Autodesk Inventor part; units mm, degrees
ref_plane "YZ Plane" through (0, 0, 0) normal (1, 0, 0) x (0, 1, 0)
ref_plane "XZ Plane" through (0, 0, 0) normal (0, 1, 0) x (-1, 0, 0)
ref_plane "XY Plane" through (0, 0, 0) normal (0, 0, 1) x (1, 0, 0)
sketch "Sketch2" plane through (0, 0, 0) normal (0, 0, 1) x (1, 0, 0)
  line L0 (-197.082, 197.082) -> (0, 278.716)
  line L1 (0, 278.716) -> (197.082, 197.082)
  line L2 (197.082, 197.082) -> (278.716, 0)
  line L3 (278.716, 0) -> (197.082, -197.082)
  line L4 (197.082, -197.082) -> (0, -278.716)
  line L5 (0, -278.716) -> (-197.082, -197.082)
  line L6 (-197.082, -197.082) -> (-278.716, 0)
  line L7 (-278.716, 0) -> (-197.082, 197.082)
  circle A0 centre (0, 0) radius 90
  dimension "d23" = 515
  dimension "d26" = 180
extrude "Plate1" add sketch "Sketch2" against normal blind 3
sketch "Sketch4" plane through (0, 0, 0) normal (0, 0, 1) x (1, 0, 0)
  circle A0 centre (0, 110) radius 6.25
  circle A1 centre (0, 0) radius 90
  circle A2 centre (0, 0) radius 110 construction
  dimension "d28" = 220
  dimension "d16" = 12.5
extrude "Extrusion1" cut sketch "Sketch4" against normal up to surface (3 mm away) contours A0
pattern_circular "Circular Pattern1" count 8 over 360 about axis through (0, 0, -10) along (0, 0, 1) of "Extrusion1"
equation "\"d23\" = Барабан_размер_по_плоскостям"
equation "\"d15\" = Thickness"
equation "\"BendRadius\" = Thickness"
equation "\"BendReliefWidth\" = Thickness"
equation "\"BendReliefDepth\" = 0.5 * Thickness"
equation "\"CornerReliefSize\" = 4 * Thickness"
equation "\"MinimumRemnant\" = 2 * Thickness"
equation "\"TransitionRadius\" = BendRadius"
equation "\"JacobiRadiusSize\" = BendRadius"
equation "\"GapSize\" = Thickness"
properties part number "DMF 01 21 Барабан торец НОС v2.1_наруж"
Geometry check sheet. Reference: the model listing, model coordinates, mm. Give positions to 0.01 mm unless a question says otherwise; leave off trailing zeros. Order: outer loops, then holes, each group sorted by start corner. A loop starts at its lowest first (then second) coordinate and runs counter-clockwise, first axis right, second up.
1. Section check D-D, the plane x = 167. Enter the section's corners in (y, z), and give its area (3 significant figures).
2. Thickness scan on L1, parallel to Y at x = 0, z = -1.8; L2, parallel to Y at x = 110.5, z = -2.7; L3, parallel to X at y = 28, z = -2.1. Record the ranges inside material, lowest first.
3. Gauge pin test, flat ends, axial feed: pin 1 Ø16 at (x, y) = (77.78, 77.78) entering from +Z; pin 2 Ø1 at (y, z) = (125, -0.5) entering from -X; pin 3 Ø1 at (y, z) = (24.5, -0.5) entering from -X. Record the tip position at first contact, or that the pin passes through.
4. Release check for a two-part mould opening along Y. For faces 1 (the face through (-97.16, -238.47, -1.48)), 2 (the face through (0.8, -116.2, -1.5)), 3 (the face through (237.328, 99.921, -1.479)), 4 (the face through (-0.8, 116.2, -1.5)) record: pulls with the +Y half, pulls with the -Y half, needs draft (parallel to the pull), parting line crosses it, or undercut.
5. Section check A-A, the plane x = 19.5. Enter the section's corners in (y, z).
6. Section check C-C, the plane y = -205. Enter the section's corners in (x, z).
7. Section check B-B, the plane z = -1.85. Give the number of separate pieces and of enclosed holes in the cut face, and give its area (3 significant figures).
Values follow:
1. outline: (-209.54, -3) - (209.54, -3) - (209.54, 0) - (-209.54, 0) - close
1. area: 1,260 mm2
2. L1: y = -278.72 to -116.25, -103.75 to -90, 90 to 103.75, 116.25 to 278.72
2. L2: y = -232.95 to -6.23, 6.23 to 232.95
2. L3: x = -267.12 to -85.53, 85.53 to 267.12
3. pin 1: stops at z = 0
3. pin 2: stops at x = -227.15
3. pin 3: stops at x = -268.77
4. face 1: pulls with the -Y half
4. face 2: undercut
4. face 3: pulls with the +Y half
4. face 4: undercut
5. outline: (-270.64, -3) - (-87.86, -3) - (-87.86, 0) - (-270.64, 0) - close; (87.86, -3) - (270.64, -3) - (270.64, 0) - (87.86, 0) - close
6. outline: (-177.97, -3) - (177.97, -3) - (177.97, 0) - (-177.97, 0) - close
7. separate pieces: 1
7. enclosed holes: 9
7. area: 193,000 mm2
